from build123d import *

# Parameters (mm, degrees)
BOSS_EXTRUDE1_DEPTH = 3
CUT_EXTRUDE1_REACH  = 122.453
SKETCH2_R           = 3.45
FILLET1_R           = 4
CUT_EXTRUDE2_REACH  = 122.453
SKETCH3_W           = 4.8
SKETCH3_H           = 3
CUT_EXTRUDE3_REACH  = 122.453
SKETCH5_R           = 1.5
BOSS_EXTRUDE2_DEPTH = 3
CUT_EXTRUDE4_REACH  = 122.453
SKETCH5_3_R         = 1.5
FILLET2_R           = 1
CUT_EXTRUDE5_REACH  = 122.453
SKETCH6_R           = 1.5
BOSS_EXTRUDE3_START = -3
SKETCH8_R           = 1.5
BOSS_EXTRUDE3_DEPTH = 3
FILLET3_R           = 2


with BuildPart() as part:
    # Sketch1 → Boss-Extrude1 (new body)
    with BuildSketch(Plane.XY):
        with BuildLine():
            Line((0, 10), (120, 10))
            Line((120, 10), (120, -10))
            Line((120, -10), (0, -10))
            ThreePointArc((0, -10), (-10, 0), (0, 10))
        make_face()
    extrude(amount=BOSS_EXTRUDE1_DEPTH)

    # Sketch2 → Cut-Extrude1 (cut, up to next)
    with BuildSketch(Plane.XY.offset(3), mode=Mode.PRIVATE) as cut_extrude1_sk1:
        Circle(SKETCH2_R)
    cut_extrude1_tool1 = extrude(cut_extrude1_sk1.sketch, amount=-CUT_EXTRUDE1_REACH, mode=Mode.PRIVATE) & part.part
    add(cut_extrude1_tool1.solids().sort_by_distance((0, 0, 3))[0], mode=Mode.SUBTRACT)

    # Fillet1
    fillet1_edges = [part.edges().sort_by_distance(p)[0] for p in [
        (120, 10, 1.5),
        (120, -10, 1.5),
    ]]
    fillet(fillet1_edges, radius=FILLET1_R)

    # Sketch3 → Cut-Extrude2 (cut, up to next)
    with BuildSketch(Plane.XY.offset(3), mode=Mode.PRIVATE) as cut_extrude2_sk1:
        with Locations((85.1, 6)):
            Rectangle(SKETCH3_W, SKETCH3_H)
    cut_extrude2_tool1 = extrude(cut_extrude2_sk1.sketch, amount=-CUT_EXTRUDE2_REACH, mode=Mode.PRIVATE) & part.part
    # Sketch3 → Cut-Extrude2 (cut, up to next)
    with BuildSketch(Plane.XY.offset(3), mode=Mode.PRIVATE) as cut_extrude2_sk2:
        with Locations((112.4, 6)):
            Rectangle(SKETCH3_W, SKETCH3_H)
    cut_extrude2_tool2 = extrude(cut_extrude2_sk2.sketch, amount=-CUT_EXTRUDE2_REACH, mode=Mode.PRIVATE) & part.part
    add(cut_extrude2_tool1.solids().sort_by_distance((85.1, 6, 3))[0], mode=Mode.SUBTRACT)
    add(cut_extrude2_tool2.solids().sort_by_distance((112.4, 6, 3))[0], mode=Mode.SUBTRACT)

    # Sketch4 → Cut-Extrude3 (cut, up to next)
    with BuildSketch(Plane.XY.offset(3), mode=Mode.PRIVATE) as cut_extrude3_sk1:
        with BuildLine():
            Line((11, 7.5), (71, 7.5))
            ThreePointArc((71, 7.5), (73.5, 5), (71, 2.5))
            Line((71, 2.5), (11, 2.5))
            ThreePointArc((11, 2.5), (8.5, 5), (11, 7.5))
        make_face()
    cut_extrude3_tool1 = extrude(cut_extrude3_sk1.sketch, amount=-CUT_EXTRUDE3_REACH, mode=Mode.PRIVATE) & part.part
    # Sketch4 → Cut-Extrude3 (cut, up to next)
    with BuildSketch(Plane.XY.offset(3), mode=Mode.PRIVATE) as cut_extrude3_sk2:
        with BuildLine():
            Line((11, -2.5), (111, -2.5))
            ThreePointArc((111, -2.5), (113.5, -5), (111, -7.5))
            Line((111, -7.5), (11, -7.5))
            ThreePointArc((11, -7.5), (8.5, -5), (11, -2.5))
        make_face()
    cut_extrude3_tool2 = extrude(cut_extrude3_sk2.sketch, amount=-CUT_EXTRUDE3_REACH, mode=Mode.PRIVATE) & part.part
    add(cut_extrude3_tool1.solids().sort_by_distance((41, 5, 3))[0], mode=Mode.SUBTRACT)
    add(cut_extrude3_tool2.solids().sort_by_distance((61, -5, 3))[0], mode=Mode.SUBTRACT)

    # Sketch5 → Boss-Extrude2 (add)
    # profile 1 of 3: a face of its own
    with BuildSketch(Plane.XY.offset(3)):
        with BuildLine():
            Line((52, 7.5), (48, 7.5))
            Line((48, 7.5), (48, 4.582575695))
            ThreePointArc((48, 4.582575695), (46.668047509, 3.728014565), (45.669872981, 2.5))
            Line((45.669872981, 2.5), (54.330127019, 2.5))
            ThreePointArc((54.330127019, 2.5), (53.331952491, 3.728014565), (52, 4.582575695))
            Line((52, 4.582575695), (52, 7.5))
        make_face()
    # profile 2 of 3: a face of its own
    with BuildSketch(Plane.XY.offset(3)):
        with BuildLine():
            Line((54.330127019, -2.5), (45.669872981, -2.5))
            ThreePointArc((45.669872981, -2.5), (46.668047509, -3.728014565), (48, -4.582575695))
            Line((48, -4.582575695), (48, -7.5))
            Line((48, -7.5), (52, -7.5))
            Line((52, -7.5), (52, -4.582575695))
            ThreePointArc((52, -4.582575695), (53.331952491, -3.728014565), (54.330127019, -2.5))
        make_face()
    # profile 3 of 3: a face of its own
    with BuildSketch(Plane.XY.offset(3)):
        with BuildLine():
            Line((54.330127019, 2.5), (45.669872981, 2.5))
            ThreePointArc((45.669872981, 2.5), (45, 0), (45.669872981, -2.5))
            Line((45.669872981, -2.5), (54.330127019, -2.5))
            ThreePointArc((54.330127019, -2.5), (55, 0), (54.330127019, 2.5))
        make_face()
        with Locations((50, 0)):
            Circle(SKETCH5_R, mode=Mode.SUBTRACT)
    extrude(amount=-BOSS_EXTRUDE2_DEPTH)

    # Sketch5<3> → Cut-Extrude4 (cut, up to next)
    with BuildSketch(Plane.XY.offset(3), mode=Mode.PRIVATE) as cut_extrude4_sk1:
        with Locations((50, 0)):
            Circle(SKETCH5_3_R)
    cut_extrude4_tool1 = extrude(cut_extrude4_sk1.sketch, amount=-CUT_EXTRUDE4_REACH, mode=Mode.PRIVATE) & part.part
    add(cut_extrude4_tool1.solids().sort_by_distance((50, 0, 3))[0], mode=Mode.SUBTRACT)

    # Fillet2
    fillet2_edges = [part.edges().sort_by_distance(p)[0] for p in [
        (52, 4.582575695, 1.5),
        (48, -4.582575695, 1.5),
        (48, -7.5, 1.5),
        (52, -7.5, 1.5),
        (52, -4.582575695, 1.5),
        (54.330127019, -2.5, 1.5),
        (52, 7.5, 1.5),
        (48, 7.5, 1.5),
        (48, 4.582575695, 1.5),
        (45.669872981, -2.5, 1.5),
        (45.669872981, 2.5, 1.5),
        (54.330127019, 2.5, 1.5),
    ]]
    fillet(fillet2_edges, radius=FILLET2_R)

    # Sketch6 → Cut-Extrude5 (cut, up to next)
    with BuildSketch(Plane(origin=(0, 0, 0), x_dir=(-1, 0, 0), z_dir=(0, 0, -1)), mode=Mode.PRIVATE) as cut_extrude5_sk1:
        with Locations((-12.45, 0)):
            Circle(SKETCH6_R)
    cut_extrude5_tool1 = extrude(cut_extrude5_sk1.sketch, amount=-CUT_EXTRUDE5_REACH, mode=Mode.PRIVATE) & part.part
    add(cut_extrude5_tool1.solids().sort_by_distance((12.45, 0, 0))[0], mode=Mode.SUBTRACT)

    # Sketch8 → Boss-Extrude3 (add)
    with BuildSketch(Plane.XY.offset(3).offset(BOSS_EXTRUDE3_START)):
        with BuildLine():
            Line((5, 16), (5, 10))
            Line((5, 10), (0, 10))
            ThreePointArc((0, 10), (-2.588190451, 9.659258263), (-5, 8.660254038))
            Line((-5, 8.660254038), (-5, 16))
            ThreePointArc((-5, 16), (0, 21), (5, 16))
        make_face()
        with Locations((0, 16)):
            Circle(SKETCH8_R, mode=Mode.SUBTRACT)
    extrude(amount=BOSS_EXTRUDE3_DEPTH)

    # Fillet3
    fillet3_edges = [part.edges().sort_by_distance(p)[0] for p in [
        (5, 10, 1.5),
        (-5, 8.660254038, 1.5),
    ]]
    fillet(fillet3_edges, radius=FILLET3_R)


solid = part.part
Can you work these out from the model? Positions are in its coordinate system, mm. A direction names the side the tool comes from. Round coordinates to 2 decimals unless told otherwise and drop trailing zeros. Loops run counter-clockwise (first coordinate to the right, second up) from the corner with the lowest first, then second, coordinate; pieces in that order, holes last. Notation, with made-up numbers: (22.5, 89) - (39.5, 89) arc R22 cw to (39.5, 98) - close; hole circle Ø1 at (48, 62). An arc over 180 degrees is marked (long way). Write item = value, one per line. Start each with the question number.
(1) If we section it at D-D (x = 12.45): Please give me the cut outline in (y, z), and give its area (3 significant figures).
(2) For faces 1 (the face through (-5, 13, 1)), 2 (the face through (28, -2.5, 2)), 3 (the face through (56, 2, 0)), which set-ups out of +Z, -Z, +X, -X, +Y, -Y let a thin tool reach every point of the face, with its end or its side?
(3) If I drill on probe 1 along Y at (x, z) = (12.45, 1.15); probe 2 along Y at (x, z) = (0, 2.4); probe 3 along Y at (x, z) = (22.5, 2.1), over which ranges is the centre line in solid material (lowest first)? Write a range as [from, to].
(4) For P1, Ø1.5, axis at x = 66.5, z = 1.5, coming from the +Y side; P2, Ø1.4, axis at y = 6, z = 1.5, coming from the -X side; P3, Ø1.8, axis at x = 12.45, y = 0, coming from the +Z side; P4, Ø1, axis at y = -6, z = 2, coming from the -X side, each with a flat end and sliding along its axis, tell me the tip position at first contact or that it passes through.
(5) If we section it at B-B (y = 0): Please give me the cut outline in (x, z).
(6) If we section it at A-A (x = 42): Please give me the cut outline in (y, z).
(7) If we section it at C-C (x = 75.5): Please give me the cut outline in (y, z), and give its area (3 significant figures).
(8) If we mould it in two halves opening along X, with no side actions, what happens to faces 4 (the face through (-0.45, 3.42, 1.52)), 5 (the face through (56, 2, 3)), 6 (the face through (120, 0, 1))? For each: released by +X, released by -X, zero draft, split by the parting line, or undercut.
Ans:
q1.outline = (-10, 0) - (-7.5, 0) - (-7.5, 3) - (-10, 3) - close; (-2.5, 0) - (-1.5, 0) - (-1.5, 3) - (-2.5, 3) - close; (1.5, 0) - (2.5, 0) - (2.5, 3) - (1.5, 3) - close; (7.5, 0) - (10, 0) - (10, 3) - (7.5, 3) - close
q1.area = 21.0 mm²
q2.face_1 = +Z, -Z, -X, +Y
q2.face_2 = +Z, -Z
q2.face_3 = -Z, +X, -X, +Y, -Y
q3.probe_1 = [-10, -7.5], [-2.5, -1.5], [1.5, 2.5], [7.5, 10]
q3.probe_2 = [-10, -3.45], [3.45, 14.5], [17.5, 21]
q3.probe_3 = [-10, -7.5], [-2.5, 2.5], [7.5, 10]
q4.P1 = 10
q4.P2 = -8.48
q4.P3 = through
q4.P4 = -8.35
q5.outline = (-10, 0) - (-3.45, 0) - (-3.45, 3) - (-10, 3) - close; (3.45, 0) - (10.95, 0) - (10.95, 3) - (3.45, 3) - close; (13.95, 0) - (48.5, 0) - (48.5, 3) - (13.95, 3) - close; (51.5, 0) - (120, 0) - (120, 3) - (51.5, 3) - close
q6.outline = (-10, 0) - (-7.5, 0) - (-7.5, 3) - (-10, 3) - close; (-2.5, 0) - (2.5, 0) - (2.5, 3) - (-2.5, 3) - close; (7.5, 0) - (10, 0) - (10, 3) - (7.5, 3) - close
q7.outline = (-10, 0) - (-7.5, 0) - (-7.5, 3) - (-10, 3) - close; (-2.5, 0) - (10, 0) - (10, 3) - (-2.5, 3) - close
q7.area = 45.0 mm²
q8.face_4 = undercut
q8.face_5 = zero draft
q8.face_6 = released by +X
